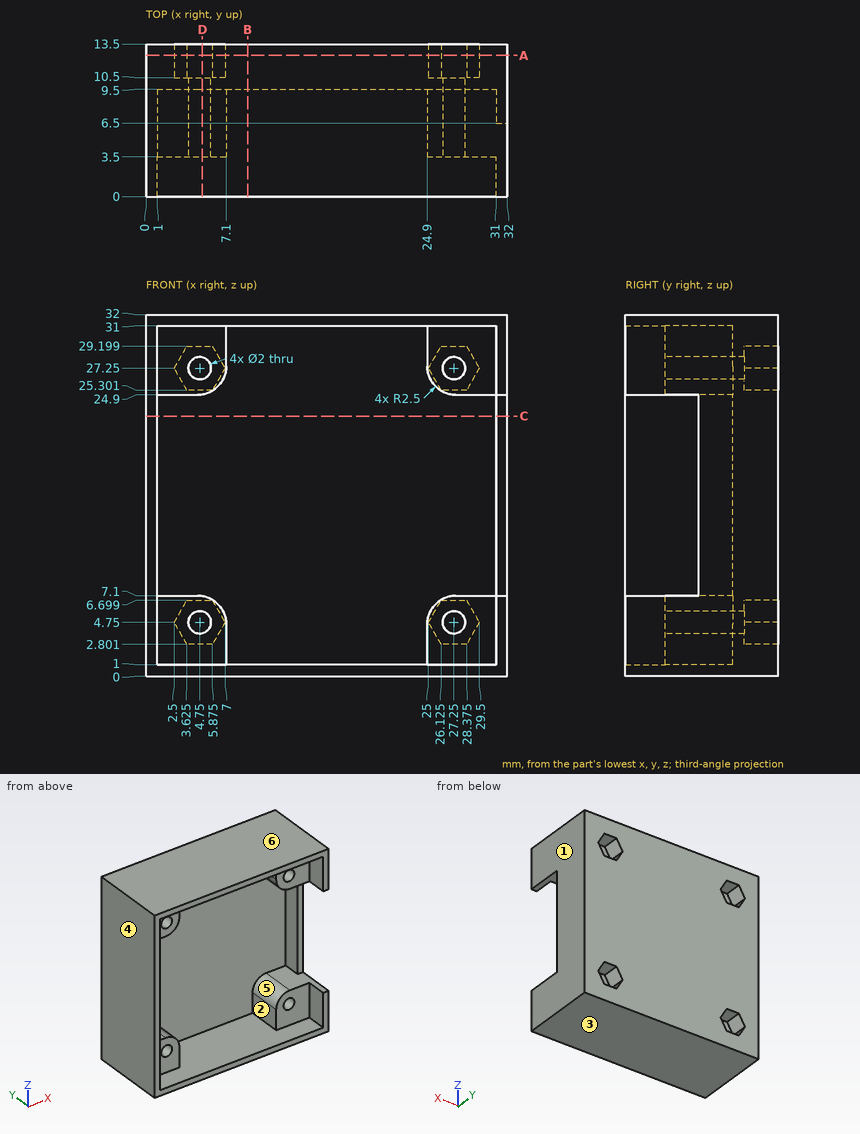
Could you check a few things on this drawing? It's one solid part, dimensions in mm from its lowest x, y, z. A direction names the side the tool comes from. Give positions to 0.01 mm unless a question says otherwise; leave off trailing zeros. Order: outer loops, then holes, each group sorted by start corner. A loop starts at its lowest first (then second) coordinate and runs counter-clockwise, first axis right, second up. Notation, with made-up numbers: (-6, 68) - (-1, 68) arc R30 cw to (-1, 105) - close; hole circle Ø3 at (38, 73). An arc over 180 degrees is marked (long way). Return JSON: item names as keys, results as strings. Group by question number.
Q1. Suppose I cut it at C-C, the plane z = 23. Please give me the cut outline in (x, y).
Q2. Suppose I cut it at D-D, the plane x = 5. Please give me the cut outline in (y, z), and give its area (3 significant figures).
Q3. Will these pins go through, and if not, where does the flat tip stop? pin 1 Ø2 at (x, y) = (23, 9.5) entering from -Z; pin 2 Ø1.8 at (x, z) = (4.75, 27.25) entering from +Y; pin 3 Ø1.9 at (x, z) = (4, 27) entering from +Y; pin 4 Ø1.8 at (x, z) = (28, 5.5) entering from -Y.
Q4. Please list where these lines run through material, in increasing order: line 1 along Z through (x, y) = (23.5, 2.75); line 2 along Y through (x, z) = (26.5, 28.5). Write a range as [from, to].
Q5. Which directions (+Z, -Z, +X, -X, +Y, -Y) give clear straight access to the entire face, cutting with the end or side of a thin tool? Please do the marked faces 1 and 2.
Q6. Suppose I cut it at B-B, the plane x = 9. Please give me the cut outline in (y, z).
Q7. Thinking about a two-plate mould opening in Z: for the marked faces 3, 4, 5 and 6, which applies, pulls with the +Z half, pulls with the -Z half, needs draft (parallel to the pull), parting line crosses it, or undercut?
Q8. Suppose I cut it at A-A, the plane y = 12.5. State how many separate pieces and enclosed holes the cut face has.
Resolved:
{
 "1": {"outline": "(0, 0) - (1, 0) - (1, 9.5) - (31, 9.5) - (31, 6.5) - (32, 6.5) - (32, 13.5) - (0, 13.5) - close"},
 "2": {"outline": "(0, 0) - (13.5, 0) - (13.5, 2.8) - (10.5, 2.8) - (10.5, 3.78) - (3.5, 3.78) - (3.5, 1) - (0, 1) - close; (0, 31) - (3.5, 31) - (3.5, 28.22) - (10.5, 28.22) - (10.5, 29.2) - (13.5, 29.2) - (13.5, 32) - (0, 32) - close; (3.5, 5.72) - (10.5, 5.72) - (10.5, 6.7) - (13.5, 6.7) - (13.5, 25.3) - (10.5, 25.3) - (10.5, 26.28) - (3.5, 26.28) - (3.5, 24.93) - (9.5, 24.93) - (9.5, 7.07) - (3.5, 7.07) - close", "area": "169 mm2"},
 "3": {"pin 1": "stops at z = 0", "pin 2": "passes through", "pin 3": "stops at y = 10.5", "pin 4": "stops at y = 3.5"},
 "4": {"line 1": "z = [0, 1], [31, 32]", "line 2": "y = [3.5, 10.5]"},
 "5": {"face 1": "+Z, -Z, +X, +Y, -Y", "face 2": "-Y"},
 "6": {"outline": "(0, 0) - (13.5, 0) - (13.5, 32) - (0, 32) - (0, 31) - (9.5, 31) - (9.5, 1) - (0, 1) - close"},
 "7": {"face 3": "pulls with the -Z half", "face 4": "needs draft", "face 5": "undercut", "face 6": "pulls with the +Z half"},
 "8": {"separate pieces": "1", "enclosed holes": "4"}
}
